Input: part model. Units: mm. Frame: model coordinates. Face numbers are marked on the shaded views. A direction names the side the tool comes from. Round coordinates to 2 decimals unless told otherwise and drop trailing zeros. Loops run counter-clockwise (first coordinate to the right, second up) from the corner with the lowest first, then second, coordinate; pieces in that order, holes last. Notation, with made-up numbers: (-31, 56.5) - (-8, 56.5) arc R22 cw to (-8, 91.5) - close; hole circle Ø4 at (-32.75, 22.25). An arc over 180 degrees is marked (long way). One line per question, with ' | ' between items. Start each with the question number.
Item 1: Section C-C, the plane y = 19.05. Return loops of the section in (x, z), plus the area to 3 significant figures.
Item 2: Section B-B, the plane y = 6.35. Return loops of the section in (x, z).
Item 3: Section D-D, the plane y = 10.25. Return loops of the section in (x, z).
Item 4: First-contact query: pin 1 (6 mm diameter, centred on x = -29.5, y = 11.5, fed in from +Z); pin 2 (4 mm diameter, centred on y = 3, z = 5.5, fed in from +X); pin 3 (2 mm diameter, centred on y = 13.16, z = 23.02, fed in from -X). Flat tips, straight axial feed; report the tip coordinate or a pass-through.
Item 5: Set-up query: the marked faces 1 and 2. Return all of +Z, -Z, +X, -X, +Y, -Y with unobstructed straight access to the full face (end or side cutting, diameter ignored); none if empty.
Item 6: Section A-A, the plane x = -21. Return loops of the section in (y, z).
Item 7: Material intervals for line 1 along X through (y, z) = (19.05, 3.95); line 2 along X through (y, z) = (23.75, 18.5); line 3 along Z through (x, y) = (-14, 12), sorted ascending.
```python
from build123d import *

# Parameters (mm, degrees)
BOSS_EXTRUDE2_DEPTH           = 25.4
TAP_DRILL_FOR_4_40_TAP1_D     = 2.2606
TAP_DRILL_FOR_4_40_TAP1_DEPTH = 3.302
TAP_DRILL_FOR_4_40_TAP1_TIP   = 0.679152758
TAP_DRILL_FOR_6_32_TAP1_D     = 2.7051
TAP_DRILL_FOR_6_32_TAP1_DEPTH = 3.302
TAP_DRILL_FOR_6_32_TAP1_TIP   = 0.81269403


with BuildPart() as part:
    # Sketch1 → Boss-Extrude2 (new body)
    with BuildSketch(Plane(origin=(0, 0, 0), x_dir=(1, 0, 0), z_dir=(0, 1, 0))):
        Polygon((-35.951603547, -27.391556999), (-32.776603547, -27.391556999), (-32.776603547, -5.166556999), (-10.551603547, -5.166556999), (-10.551603547, -1.991556999), (-35.951603547, -1.991556999), align=None)
    extrude(amount=BOSS_EXTRUDE2_DEPTH)

    # Tap Drill for #4-40 Tap1
    with Locations(Plane.ZY.offset(35.951603547)):
        with Locations((16.520356999, 19.7104), (23.022756999, 13.1572)):
            Hole(TAP_DRILL_FOR_4_40_TAP1_D / 2, depth=TAP_DRILL_FOR_4_40_TAP1_DEPTH)
            with Locations((0, 0, -(TAP_DRILL_FOR_4_40_TAP1_DEPTH + TAP_DRILL_FOR_4_40_TAP1_TIP / 2))):  # 118° drill point
                Cone(0, TAP_DRILL_FOR_4_40_TAP1_D / 2, TAP_DRILL_FOR_4_40_TAP1_TIP, mode=Mode.SUBTRACT)

    # Tap Drill for #6-32 Tap1
    with Locations(Plane(origin=(-21.664103547, 6.35, 5.166556999), x_dir=(1, 0, 0), z_dir=(0, 0, 1))):
        with Locations((0, 0), (0.113463967, 12.7)):
            Hole(TAP_DRILL_FOR_6_32_TAP1_D / 2, depth=TAP_DRILL_FOR_6_32_TAP1_DEPTH)
            with Locations((0, 0, -(TAP_DRILL_FOR_6_32_TAP1_DEPTH + TAP_DRILL_FOR_6_32_TAP1_TIP / 2))):  # 118° drill point
                Cone(0, TAP_DRILL_FOR_6_32_TAP1_D / 2, TAP_DRILL_FOR_6_32_TAP1_TIP, mode=Mode.SUBTRACT)


solid = part.part
```
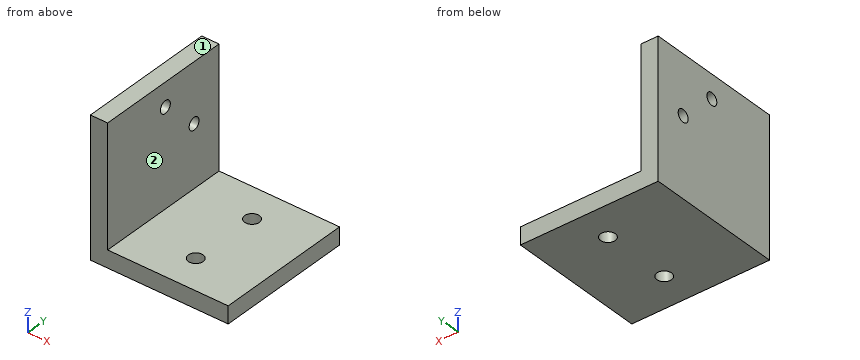
Return value:
1) outline: (-35.95, 1.99) - (-22.9, 1.99) - (-22.9, 5.17) - (-32.78, 5.17) - (-32.78, 15.6) - (-35.95, 15.6) - close; (-35.95, 17.44) - (-32.78, 17.44) - (-32.78, 27.39) - (-35.95, 27.39) - close; (-20.2, 1.99) - (-10.55, 1.99) - (-10.55, 5.17) - (-20.2, 5.17) - close | area: 137 mm2
2) outline: (-35.95, 1.99) - (-23.02, 1.99) - (-23.02, 5.17) - (-32.78, 5.17) - (-32.78, 27.39) - (-35.95, 27.39) - close; (-20.31, 1.99) - (-10.55, 1.99) - (-10.55, 5.17) - (-20.31, 5.17) - close
3) outline: (-35.95, 1.99) - (-10.55, 1.99) - (-10.55, 5.17) - (-32.78, 5.17) - (-32.78, 27.39) - (-35.95, 27.39) - close
4) pin 1: z = 5.17 | pin 2: x = -10.55 | pin 3: through
5) face 1: +Z, +X, -X, +Y, -Y | face 2: +Z, +X, +Y, -Y
6) outline: (0, 1.99) - (5.17, 1.99) - (5.17, 5.17) - (0, 5.17) - close; (7.53, 1.99) - (17.81, 1.99) - (17.81, 5.17) - (7.53, 5.17) - close; (20.29, 1.99) - (25.4, 1.99) - (25.4, 5.17) - (20.29, 5.17) - close
7) line 1: -35.95 to -22.9, -20.2 to -10.55 | line 2: -35.95 to -32.78 | line 3: 1.99 to 5.17
